Autodesk Fusion 360 part; units mm, degrees
sketch "Sketch1" plane through (0, 0, 0) normal (0, 0, 1) x (1, 0, 0)
  line L0 (-13.9084, 7.56) -> (36.9716, 7.56)
  line L1 (36.9716, 7.56) -> (36.9716, 25.03)
  line L2 (36.9716, 25.03) -> (-13.9084, 25.03)
  line L3 (-13.9084, 25.03) -> (-13.9084, 7.56)
  line L4 (-13.9084, 7.56) -> (-2.9084, 7.56) construction
  line L5 (36.9716, 7.56) -> (25.9716, 7.56) construction
  dimension "d4" = 50.88
  dimension "d5" = 17.47
  dimension "d7" = 11
  dimension "d8" = 11
sketch "Sketch2" plane through (0, 0, 0) normal (0, 0, 1) x (1, 0, 0)
  line L0 (11.5316, 0) -> (29.1316, 0)
  line L1 (11.5316, 0) -> (-6.0684, 0)
  line L2 (-13.9084, 7.56) -> (36.9716, 7.56)
  line L3 (-2.9084, 7.56) -> (-6.0684, 0)
  line L4 (25.9716, 7.56) -> (29.1316, 0)
  point P0 (-2.9084, 7.56)
  point P1 (25.9716, 7.56)
  dimension "d9" = 17.6
  dimension "d10" = 17.6
  dimension "d11" = 7.56
extrude "Extrude1" add sketch "Sketch1" sketch "Sketch2" along normal blind 19.16 of sketch 2
sketch "Sketch4" plane through (0, 0, 0) normal (0, 1, 0) x (1, 0, 0)
  circle A0 centre (2.9316, -9.8352) radius 6.57
  line L0 (-6.0684, 0) -> (-6.0684, -19.16)
  circle A1 centre (20.1316, -9.8352) radius 6.57
  line L1 (29.1316, 0) -> (29.1316, -19.16)
  line L2 (2.9316, -16.4052) -> (20.1316, -16.4052)
  line L3 (2.9387, -3.2652) -> (20.1316, -3.2652)
  dimension "d14" = 13.14
  dimension "d16" = 13.14
  dimension "d17" = 9
  dimension "d18" = 9
extrude "Extrude2" cut sketch "Sketch4" along normal blind 5
sketch "Sketch5" plane through (0, 25.03, 0) normal (0, 1, 0) x (-1, 0, 0)
  line L0 (-36.9716, 0) -> (13.9084, 0)
  line L1 (13.9084, 0) -> (13.9084, 19.16)
  line L2 (13.9084, 19.16) -> (-36.9716, 19.16)
  line L3 (-36.9716, 19.16) -> (-36.9716, 0)
  circle A0 centre (-20.1316, 9.58) radius 6.5
  circle A1 centre (-1.8809, 9.58) radius 6.5
  circle A2 centre (-20.1316, 9.58) radius 4
  circle A3 centre (-1.8809, 9.58) radius 4
  dimension "d21" = 13
  dimension "d22" = 13
  dimension "d24" = 9.58
  dimension "d25" = 9.58
  dimension "d26" = 8
  dimension "d27" = 8
extrude "Extrude3" cut sketch "Sketch5" against normal blind 5 contours A0 | A1
extrude "Extrude4" cut 2 faces at (2.6679, 25.03, 7.9458) (19.0151, 25.03, 9.0276) along direction (0, 1, 0) up to surface end surface through (0, 5, 0) normal (0, -1, 0) offset 0
equation "d12 = thickness"
equation "d19 = boltSink"
equation "d21 = boltH"
equation "d22 = boltH"
equation "thickness = 19.16 mm"
equation "d24 = ( 19.16 / 2 ) * 1 mm"
equation "d26 = bolt"
equation "d27 = bolt"
equation "boltH = 13 mm"
equation "boltSink = 5 mm"
equation "bolt = 8 mm"
Source: CAD feature listing. Evaluate the final solid. Frame: model axes, mm. A direction names the side the tool comes from. Round coordinates to 2 decimals unless told otherwise and drop trailing zeros. Loops run counter-clockwise (first coordinate to the right, second up) from the corner with the lowest first, then second, coordinate; pieces in that order, holes last.
Q1. Section A-A, the plane x = 22.5. Return loops of the section in (y, z).
Q2. Ray query, line 1 (X direction, y = 22.5, z = 9.5); line 2 (Y direction, x = -1, z = 13.25); line 3 (X direction, y = 5.5, z = 13.25). Return the intervals inside material, ascending.
Q3. Access query for faces 1 (the face through (26.7, 2.5, 9.7)), 2 (the face through (-1, 20.03, 13)), 3 (the face through (-8, 7.56, 9)). Directions: +Z, -Z, +X, -X, +Y, -Y. A direction counts if a zero-diameter tool reaches every point of the face in a straight line with its end or side. Return the directions, or none.
Q4. Mould query, pull axis X, two halves, no side actions, for faces 4 (the face through (-4.466, 3.833, 9.446)), 5 (the face through (31, 7.56, 9)), 6 (the face through (-3.637, 2.465, 9.976)). Classes: pulls with the +X half, pulls with the -X half, needs draft (parallel to the pull), parting line crosses it, or undercut.
Q5. Section D-D, the plane y = 22. Return loops of the section in (x, z), plus the area to 3 significant figures.
Q6. First-contact query: P1, Ø9, axis at x = 20.13, z = 9.58, coming from the +Y side; P2, Ø3.5, axis at x = -8.5, z = 12, coming from the -Y side; P3, Ø8, axis at x = 10, z = 8, coming from the -Y side. Flat tips, straight axial feed; report the tip coordinate or a pass-through.
Q7. Section C-C, the plane z = 9.58. Return loops of the section in (x, y), plus the area to 3 significant figures.
Q8. Section B-B, the plane z = 1.5. Return loops of the section in (x, y).
Solutions:
1. outline: (0, 0) - (25.03, 0) - (25.03, 3.53) - (20.03, 3.53) - (20.03, 6.36) - (5, 6.36) - (5, 3.71) - (0, 3.71) - close; (0, 15.96) - (5, 15.96) - (5, 12.8) - (20.03, 12.8) - (20.03, 15.63) - (25.03, 15.63) - (25.03, 19.16) - (0, 19.16) - close
2. line 1: x = -13.91 to -4.62, 8.38 to 13.63, 26.63 to 36.97
2. line 2: y = 5 to 20.03
2. line 3: x = -3.77 to 0.29, 3.47 to 18.54, 21.72 to 26.83
3. face 1: -Y
3. face 2: +Y
3. face 3: +Z, -Z, -X
4. face 4: pulls with the -X half
4. face 5: needs draft
4. face 6: undercut
5. outline: (-13.91, 0) - (36.97, 0) - (36.97, 19.16) - (-13.91, 19.16) - close; hole circle Ø13 at (1.88, 9.58); hole circle Ø13 at (20.13, 9.58)
5. area: 709 mm2
6. P1: stops at y = 20.03
6. P2: stops at y = 7.56
6. P3: stops at y = 5
7. outline: (-13.91, 7.56) - (-2.91, 7.56) - (-6.07, 0) - (-3.63, 0) - (-3.63, 5) - (-2.12, 5) - (-2.12, 20.03) - (-4.62, 20.03) - (-4.62, 25.03) - (-13.91, 25.03) - close; (5.88, 5) - (16.13, 5) - (16.13, 20.03) - (13.63, 20.03) - (13.63, 25.03) - (8.38, 25.03) - (8.38, 20.03) - (5.88, 20.03) - close; (24.13, 5) - (26.7, 5) - (26.7, 0) - (29.13, 0) - (25.97, 7.56) - (36.97, 7.56) - (36.97, 25.03) - (26.63, 25.03) - (26.63, 20.03) - (24.13, 20.03) - close
7. area: 609 mm2
8. outline: (-13.91, 7.56) - (-2.91, 7.56) - (-6.07, 0) - (29.13, 0) - (25.97, 7.56) - (36.97, 7.56) - (36.97, 25.03) - (-13.91, 25.03) - close
